```python
from build123d import *

# Parameters (mm, degrees)
ESQUISSE1_R        = 15
BOSS_EXTRU_1_DEPTH = 15
CONG_1_R           = 10
ESQUISSE3_R        = 10
BOSS_EXTRU_3_DEPTH = 70


with BuildPart() as part:
    # Esquisse1 → Boss.-Extru.1 (new body)
    with BuildSketch(Plane(origin=(0, 0, 0), x_dir=(1, 0, 0), z_dir=(0, 1, 0))):
        Circle(ESQUISSE1_R)
    extrude(amount=BOSS_EXTRU_1_DEPTH)

    # Congé1
    cong_1_edges = [part.edges().sort_by_distance(p)[0] for p in [
        (-15, 15, 0),
    ]]
    fillet(cong_1_edges, radius=CONG_1_R)

    # Esquisse3 → Boss.-Extru.3 (add)
    with BuildSketch(Plane.XZ):
        Circle(ESQUISSE3_R)
    extrude(amount=BOSS_EXTRU_3_DEPTH)


solid = part.part
```
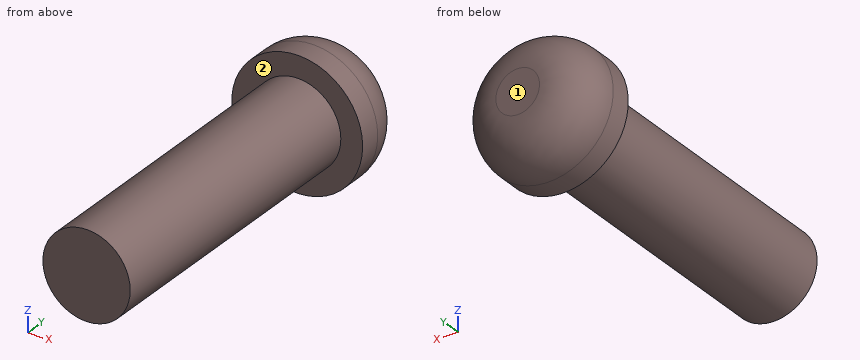
CAD build for the part. Positions are in the model's coordinates, mm. Face numbers are marked on the shaded views. A direction names the side the tool comes from. Round coordinates to 2 decimals unless told otherwise and drop trailing zeros. Order: outer loops, then holes, each group sorted by start corner. A loop starts at its lowest first (then second) coordinate and runs counter-clockwise, first axis right, second up.
Item 1: Tool access for the marked faces 1 and 2: list every direction of +Z, -Z, +X, -X, +Y, -Y with a clear straight run to the whole face (end or side of a thin tool).
Item 2: Probe line 1 along X through (y, z) = (6, -9); line 2 along Y through (x, z) = (-6.25, -12.75); line 3 along Y through (x, z) = (0.75, -11.75). List the from-to ranges inside material, lowest first.
Item 3: Saw through at A-A on y = -50. Write the cut outline in (x, z), then the cut area to 3 significant figures.
Item 4: Pin check, flat tips, straight feed: pin 1 (12 mm diameter, centred on y = 4, z = 9, fed in from -X); pin 2 (4 mm diameter, centred on y = -23.5, z = 10.5, fed in from +X); pin 3 (3 mm diameter, centred on y = -51, z = -10.5, fed in from -X); pin 4 (1.5 mm diameter, centred on y = -20, z = 11, fed in from -X). Stop position of each tip, or through.
Reported:
1. face 1: +Z, -Z, +X, -X, +Y
1. face 2: -Y
2. line 1: x = -11.94 to 11.94
2. line 2: y = 0 to 8.92
2. line 3: y = 0 to 12.36
3. outline: circle Ø20 at (0, 0)
3. area: 314 mm2
4. pin 1: stops at x = -14.7
4. pin 2: stops at x = 5.27
4. pin 3: stops at x = -4.36
4. pin 4: passes through
